Work out the finished part from the listing and answer in its coordinate system (mm). Face numbers are marked on the shaded views. A direction names the side the tool comes from. Round coordinates to 2 decimals unless told otherwise and drop trailing zeros. Loops run counter-clockwise (first coordinate to the right, second up) from the corner with the lowest first, then second, coordinate; pieces in that order, holes last.
```python
from build123d import *

# Parameters (mm, degrees)
F1_DEPTH = 30
F2_R     = 10
F3_R     = 5
F4_R     = 12
F5_R     = 10
F7_D     = 5
F8_T     = -2.5


with BuildPart() as f1:
    # F0 (on Top) → F1 (new body)
    with BuildSketch(Plane.XY):
        with BuildLine():
            Line((15.899289, 61.283179), (-15.899289, 61.283179))
            Line((-15.899289, 61.283179), (-21.571181, 25.174486))
            Line((-21.571181, 25.174486), (-35, 20))
            Line((-35, 20), (-35, 0))
            ThreePointArc((-35, 0), (0, -35), (35, 0))
            Line((35, 0), (35, 20))
            Line((35, 20), (21.571181, 25.174486))
            Line((21.571181, 25.174486), (15.899289, 61.283179))
        make_face()
    extrude(amount=F1_DEPTH)

    # F2
    f2_edges = [f1.edges().sort_by_distance(p)[0] for p in [
        (35, 20, 15),
        (-35, 20, 15),
    ]]
    fillet(f2_edges, radius=F2_R)

    # F3
    f3_edges = [f1.edges().sort_by_distance(p)[0] for p in [
        (21.571181, 25.174486, 15),
        (-21.571181, 25.174486, 15),
    ]]
    fillet(f3_edges, radius=F3_R)

    # F4
    f4_edges = [f1.edges().sort_by_distance(p)[0] for p in [
        (15.899289, 61.283179, 15),
        (-15.899289, 61.283179, 15),
    ]]
    fillet(f4_edges, radius=F4_R)

    # F5
    f5_edges = [f1.edges().sort_by_distance(p)[0] for p in [
        (19.30748, 39.585778, 0),
    ]]
    fillet(f5_edges, radius=F5_R)

    # F7 (through all)
    with Locations(Plane.XY.offset(30)):
        with Locations((0, 50.086495)):
            Hole(F7_D / 2)

    # F8
    f8_openings = [f1.faces().sort_by_distance(p)[0] for p in [
        (0, 9.29282, 30),
    ]]
    offset(amount=F8_T, openings=f8_openings)


solid = f1.part
```
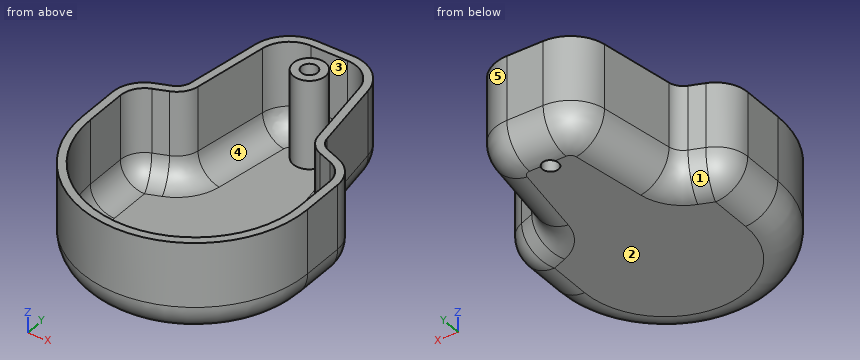
1. Given pin 1 (4 mm diameter, centred on y = -3, z = 3, fed in from +X); pin 2 (3 mm diameter, centred on x = 15.5, z = 15, fed in from -Y); pin 3 (12 mm diameter, centred on y = -10, z = 17.5, fed in from +X); pin 4 (3 mm diameter, centred on x = 21.5, y = 45.5, fed in from -Z), each flat-ended and moving along its own axis, determine where each tip first touches the part or whether it passes through.
Answer key:
pin 1: stops at x = 33.54
pin 2: stops at y = -32.08
pin 3: stops at x = 34.77
pin 4: passes through
2. Determine the mould class of the marked faces 1, 2 and 3 for opening direction Y: +Y half, -Y half, draft (parallel to the pull), parting line (faces both ways), or undercut.
Answer key:
face 1: +Y half
face 2: draft
face 3: undercut
3. Consider probe 1 along Y at (x, z) = (0, 9.5); probe 2 along Y at (x, z) = (0, 9); probe 3 along X at (y, z) = (50, 10.5). Determine where each line is inside the solid, lowest interval first.
Answer key:
probe 1: y = -34.99 to -32.48, 45.09 to 47.59, 52.59 to 55.09, 58.77 to 61.27
probe 2: y = -34.95 to -32.43, 45.09 to 47.59, 52.59 to 55.09, 58.72 to 61.23
probe 3: x = -17.67 to -15.14, -5 to -2.5, 2.5 to 5, 15.14 to 17.67
4. Find section B-B (x = 0). Write down the section's boundary in (y, z), then the cut area to 3 significant figures.
Answer key:
outline: (-35, 10) arc R10 ccw to (-25, 0) - (47.59, 0) - (47.59, 30) - (45.09, 30) - (45.09, 2.5) - (-25, 2.5) arc R7.5 cw to (-32.5, 10) - (-32.5, 30) - (-35, 30) - close; (52.59, 0.09) arc R10 ccw to (61.28, 10) - (61.28, 30) - (58.78, 30) - (58.78, 10) arc R7.5 cw to (55.09, 3.54) - (55.09, 30) - (52.59, 30) - close
area: 483 mm2
5. Which of the six approach directions +Z, -Z, +X, -X, +Y, -Y give full straight-line access (tool end or side, diameter ignored) to the marked faces 4 and 5?
Answer key:
face 4: +Z
face 5: +Z, -Z, +X, +Y
6. Find section A-A (z = 22). Give the number of separate pieces and of enclosed holes in the cut face, then the cut area to 3 significant figures.
Answer key:
separate pieces: 2
enclosed holes: 2
area: 719 mm2
